Verification items for the finished model (mm, model axes). Face numbers are marked on the shaded views. A direction names the side the tool comes from. Coordinates: 2 decimals unless noted, no trailing zeros. Order: outer loops, then holes, each group sorted by start corner. A loop starts at its lowest first (then second) coordinate and runs counter-clockwise, first axis right, second up. Notation, with made-up numbers: M 44,30 L 77,30 A18 ccw 77,48 Z; hole C 8.25,-29.5 d4. An arc over 180 degrees is marked long. Use one line per item in the form item = value. Start each with the question number.
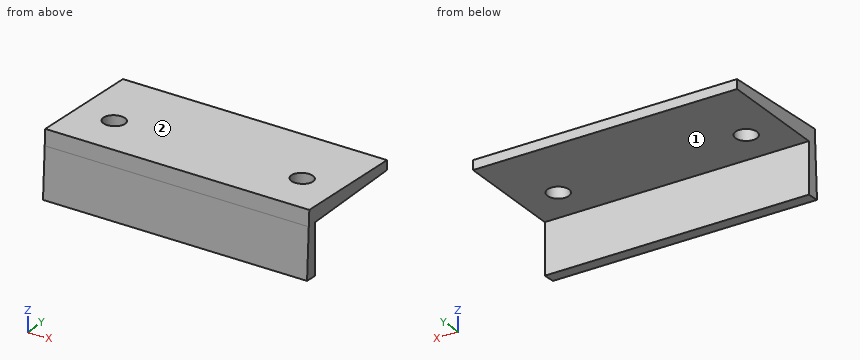
```python
from build123d import *

# Parameters (mm, degrees)
SKETCH1_W           = 84
SKETCH1_H           = 38
BOSS_EXTRUDE1_DEPTH = 5
SKETCH2_W           = 84
SKETCH2_H           = 42
CUT_REVOLVE1_ANGLE  = 3
SKETCH5_W           = 84
SKETCH5_H           = 5
REVOLVE1_ANGLE      = 3
BOSS_EXTRUDE3_DEPTH = 84
SKETCH4_R           = 3.4
CUT_EXTRUDE1_DEPTH  = 10


with BuildPart() as part:
    # Sketch1 → Boss-Extrude1 (new body)
    with BuildSketch(Plane.XY):
        Rectangle(SKETCH1_W, SKETCH1_H)
    extrude(amount=BOSS_EXTRUDE1_DEPTH)

    # Sketch2 → Cut-Revolve1 (revolve, cut)
    with BuildSketch(Plane.XY.offset(5)):
        with Locations((0, 2)):
            Rectangle(SKETCH2_W, SKETCH2_H)
    revolve(axis=Axis((-42, -19, 5), (-1, 0, 0)), revolution_arc=CUT_REVOLVE1_ANGLE, mode=Mode.SUBTRACT)

    # Sketch5 → Revolve1 (revolve)
    with BuildSketch(Plane.XZ.offset(19)):
        with Locations((0, 2.5)):
            Rectangle(SKETCH5_W, SKETCH5_H)
    revolve(axis=Axis((-42, -19, 5), (-1, 0, 0)), revolution_arc=REVOLVE1_ANGLE)

    # Sketch6 → Boss-Extrude3 (add)
    with BuildSketch(Plane(origin=(-42, 0, 0), x_dir=(0, -1, 0), z_dir=(-1, 0, 0))):
        Polygon((19.261679781, 0.006852326), (20.10020425, -15.993147674), (16.10020425, -16.202778791), (16.10020425, 0), align=None)
    extrude(amount=-BOSS_EXTRUDE3_DEPTH)

    # Sketch4 → Cut-Extrude1 (cut)
    with BuildSketch(Plane(origin=(0, 0.209279164, 3.993284337), x_dir=(1, 0, 0), z_dir=(0, 0.052335956, 0.998629535))):
        with Locations((29.895651858, -4.083491794)):
            Circle(SKETCH4_R)
        with Locations((-29.895651858, -4.083491794)):
            Circle(SKETCH4_R)
    extrude(amount=-CUT_EXTRUDE1_DEPTH, mode=Mode.SUBTRACT)


solid = part.part
```
1. Depth check by flat-ended pin: P1, Ø3, axis at x = 28.5, z = -10, coming from the +Y side; P2, Ø3, axis at x = -28, y = 3, coming from the -Z side; P3, Ø5, axis at x = -4, z = -9.5, coming from the -Y side. Enter the tip coordinate at first touch or a pass-through.
2. Cross-section at C-C on z = -12.75. Enter the section's corners in (x, y), and give its area (3 significant figures).
3. Cross-section at A-A on x = -28. Enter the section's corners in (y, z), and give its area (3 significant figures).
4. Cross-section at B-B on x = -5.5. Enter the section's corners in (y, z).
5. Tool access check on the marked faces 1 and 2. Record the directions out of +Z, -Z, +X, -X, +Y, -Y that give a thin tool (end or side, any length) a straight path to the whole face; none if there is none.
6. Material ranges on line 1 along Y through (x, z) = (-31.5, -0.25); line 2 along Z through (x, y) = (12, 8.5); line 3 along Y through (x, z) = (-13, -14.25), recorded low to high.
7. Cross-section at D-D on y = -5.5. Give the number of separate pieces and of enclosed holes in the cut face, and give its area (3 significant figures).
Final values:
q1.P1 = -16.1
q1.P2 = 0
q1.P3 = -19.89
q2.outline = M -42,-19.93 L 42,-19.93 L 42,-16.1 L -42,-16.1 Z
q2.area = 322 mm2
q3.outline = M -20.1,-15.99 L -16.1,-16.2 L -16.1,0 L -6.92,0 L -6.69,4.35 L -19,5 Z; M -1.26,0 L 19,0 L 19,3.01 L -1.05,4.06 Z
q3.area = 187 mm2
q4.outline = M -20.1,-15.99 L -16.1,-16.2 L -16.1,0 L 19,0 L 19,3.01 L -19,5 Z
q5.face_1 = -Z, +X, -X, +Y
q5.face_2 = +Z, +X, -X, +Y
q6.line_1 = -19.28 to -16.1
q6.line_2 = 0 to 3.56
q6.line_3 = -20.01 to -16.1
q7.separate_pieces = 3
q7.enclosed_holes = 0
q7.area = 308 mm2
